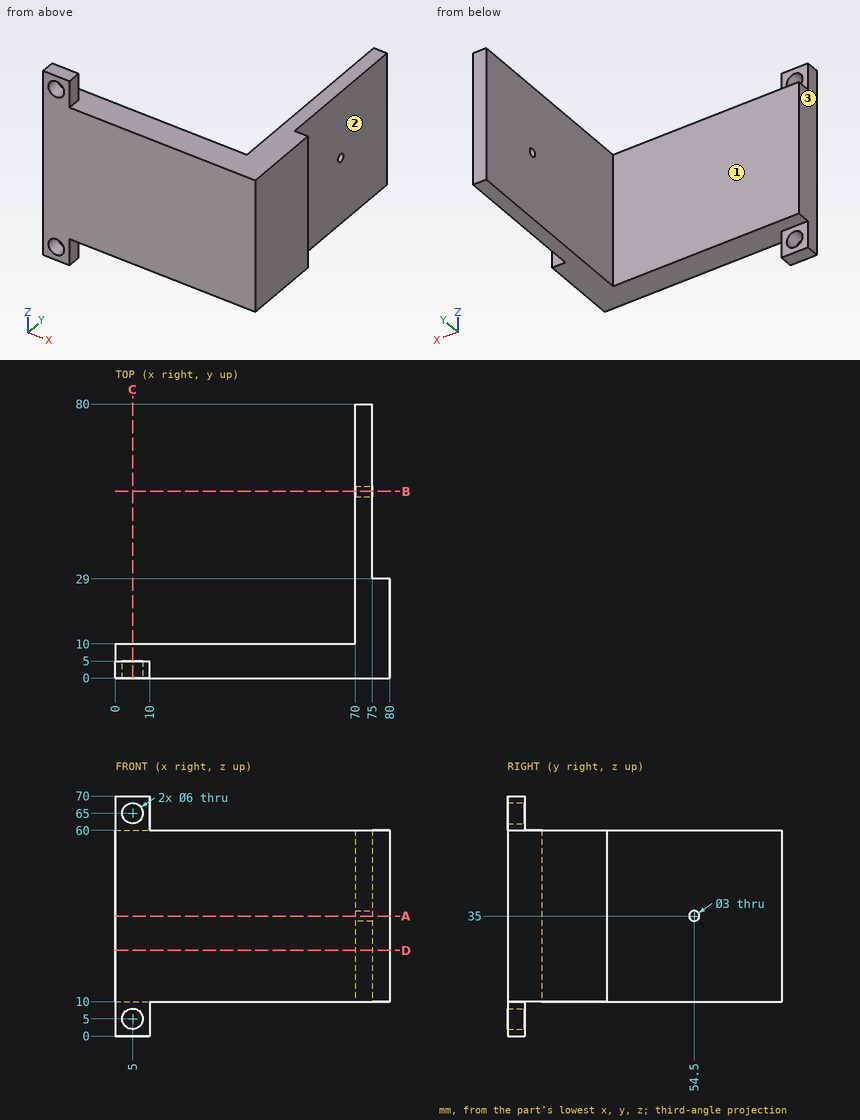
Here's the drawing with two shaded views (mm, measured from the low corner). I have some questions. A direction names the side the tool comes from. Round coordinates to 2 decimals unless told otherwise and drop trailing zeros. Loops run counter-clockwise (first coordinate to the right, second up) from the corner with the lowest first, then second, coordinate; pieces in that order, holes last. Notation, with made-up numbers: M -27.75,56 L 21.25,56 A16 cw 21.25,83 Z; hole C -38,7.25 d4. An arc over 180 degrees is marked long. Answer as a JSON object with one key per item and string values. Group by question number.
Q1. Imagine slicing it at D-D, the plane z = 25. Please give me the cut outline in (x, y), then the cut area to 4 significant figures.
Q2. Please list where these lines run through material, in increasing order: L1, parallel to Z at x = 5, y = 1.25; L2, parallel to X at y = 2, z = 65; L3, parallel to Y at x = 16, z = 26.5.
Q3. On a 3-axis mill with a long thin cutter (end or side, diameter ignored), from which of +Z, -Z, +X, -X, +Y, -Y can I reach the whole of each face in a straight line? I mean the marked faces 1, 2 and 3. Say none if no direction works.
Q4. Will these pins go through, and if not, where does the flat tip stop? pin 1 (1 mm diameter, centred on x = 46, z = 16, fed in from +Y); pin 2 (1.5 mm diameter, centred on x = 78.5, z = 26, fed in from +Y); pin 3 (3 mm diameter, centred on x = 6, z = 4.5, fed in from +Y); pin 4 (3 mm diameter, centred on x = 7.5, z = 65, fed in from +Y).
Q5. Imagine slicing it at B-B, the plane y = 54.5. Please give me the cut outline in (x, z).
Q6. Imagine slicing it at C-C, the plane x = 5. Please give me the cut outline in (y, z).
Q7. Imagine slicing it at A-A, the plane z = 35. Please give me the cut outline in (x, y), then the cut area to 3 significant figures.
Findings:
{
 "1": {"outline": "M 0,0 L 80,0 L 80,29 L 75,29 L 75,80 L 70,80 L 70,10 L 0,10 Z", "area": "1,245 mm2"},
 "2": {"L1": "z = 0 to 2, 8 to 62, 68 to 70", "L2": "x = 0 to 2, 8 to 10", "L3": "y = 0 to 10"},
 "3": {"face 1": "+Z, -Z, -X, +Y", "face 2": "+Z, -Z, +X, +Y", "face 3": "+Z, -Z, -X, +Y, -Y"},
 "4": {"pin 1": "stops at y = 10", "pin 2": "stops at y = 29", "pin 3": "passes through", "pin 4": "stops at y = 5"},
 "5": {"outline": "M 70,10 L 75,10 L 75,33.5 L 70,33.5 Z; M 70,36.5 L 75,36.5 L 75,60 L 70,60 Z"},
 "6": {"outline": "M 0,0 L 5,0 L 5,2 L 0,2 Z; M 0,8 L 5,8 L 5,10 L 10,10 L 10,60 L 5,60 L 5,62 L 0,62 Z; M 0,68 L 5,68 L 5,70 L 0,70 Z"},
 "7": {"outline": "M 0,0 L 80,0 L 80,29 L 75,29 L 75,53 L 70,53 L 70,10 L 0,10 Z; M 70,56 L 75,56 L 75,80 L 70,80 Z", "area": "1,230 mm2"}
}
